Geometry: final body of the model. Coordinates: model frame, mm. Give positions to 0.01 mm unless a question says otherwise; leave off trailing zeros. Order: outer loops, then holes, each group sorted by start corner. A loop starts at its lowest first (then second) coordinate and runs counter-clockwise, first axis right, second up. Notation, with made-up numbers: (73, 77) - (131, 77) arc R34 ccw to (131, 109) - close; hole circle Ø3 at (1, -9). An arc over 180 degrees is marked (long way). Use one line per item in the form item = value.
Autodesk Inventor part; units mm, degrees
ref_plane "YZ Plane" through (0, 0, 0) normal (1, 0, 0) x (0, 1, 0)
ref_plane "XZ Plane" through (0, 0, 0) normal (0, 1, 0) x (-1, 0, 0)
ref_plane "XY Plane" through (0, 0, 0) normal (0, 0, 1) x (1, 0, 0)
ref_plane "Work Plane1" through (0, 0, 0) normal (0, 0, 1) x (1, 0, 0)
sketch "Sketch1" plane through (0, 0, 0) normal (0, 0, 1) x (1, 0, 0)
  line L0 (468.9048, -89.2586) -> (468.9048, 5.0009)
  arc A0 (468.9048, 5.0009) -> (465.7298, 8.1759) centre (465.7298, 5.0009) ccw
  line L1 (465.7298, 8.1759) -> (360.311, 8.1759)
  line L2 (458.2368, -92.4336) -> (458.2368, -2.4921)
  line L3 (458.2368, -2.4921) -> (357.136, -2.4921)
  arc A1 (360.311, 8.1759) -> (357.136, 5.0009) centre (360.311, 5.0009) ccw
  line L4 (357.136, 5.0009) -> (357.136, -89.2586)
  arc A2 (357.136, -89.2586) -> (360.311, -92.4336) centre (360.311, -89.2586) ccw
  line L5 (360.311, -92.4336) -> (465.7298, -92.4336)
  arc A3 (465.7298, -92.4336) -> (468.9048, -89.2586) centre (465.7298, -89.2586) ccw
  line L6 (468.9048, -89.2586) -> (468.9048, 5.0009)
  arc A4 (468.9048, 5.0009) -> (465.7298, 8.1759) centre (465.7298, 5.0009) ccw
  line L7 (465.7298, 8.1759) -> (360.311, 8.1759)
  circle A5 centre (437.65, 3.8619) radius 2.5844
  circle A6 centre (372.6092, -23.0789) radius 2.5844
  circle A7 centre (399.55, -88.1196) radius 2.5844
  circle A8 centre (464.5908, -61.1789) radius 2.5844
  circle A9 centre (372.6092, -88.1196) radius 2.413
  circle A10 centre (412.25, 3.8619) radius 2.413
  circle A11 centre (464.5908, -73.8789) radius 2.413
  circle A12 centre (464.5908, -48.4789) radius 2.413
  circle A13 centre (464.5908, -35.7789) radius 2.413
  circle A14 centre (374.15, 3.8619) radius 2.413
  circle A15 centre (386.85, 3.8619) radius 2.413
  arc A16 (365.5823, -19.7251) -> (365.5823, -17.8759) centre (362.2803, -18.8005) ccw
  line L8 (365.5823, -19.7251) -> (365.5823, -22.1025)
  line L9 (365.5823, -22.1025) -> (363.2049, -22.1025)
  arc A17 (361.3557, -22.1025) -> (363.2049, -22.1025) centre (362.2803, -18.8005) ccw
  line L10 (361.3557, -22.1025) -> (358.9783, -22.1025)
  line L11 (358.9783, -22.1025) -> (358.9783, -19.7251)
  arc A18 (358.9783, -17.8759) -> (358.9783, -19.7251) centre (362.2803, -18.8005) ccw
  line L12 (358.9783, -17.8759) -> (358.9783, -15.4985)
  line L13 (358.9783, -15.4985) -> (361.3557, -15.4985)
  arc A19 (363.2049, -15.4985) -> (361.3557, -15.4985) centre (362.2803, -18.8005) ccw
  line L14 (363.2049, -15.4985) -> (365.5823, -15.4985)
  line L15 (365.5823, -15.4985) -> (365.5823, -17.8759)
  circle A20 centre (424.95, 3.8619) radius 2.413
  arc A21 (358.9783, -64.5327) -> (358.9783, -66.3818) centre (362.2803, -65.4572) ccw
  line L16 (358.9783, -64.5327) -> (358.9783, -62.1552)
  line L17 (358.9783, -62.1552) -> (361.3557, -62.1552)
  arc A22 (363.2049, -62.1552) -> (361.3557, -62.1552) centre (362.2803, -65.4572) ccw
  line L18 (363.2049, -62.1552) -> (365.5823, -62.1552)
  line L19 (365.5823, -62.1552) -> (365.5823, -64.5327)
  arc A23 (365.5823, -66.3818) -> (365.5823, -64.5327) centre (362.2803, -65.4572) ccw
  line L20 (365.5823, -66.3818) -> (365.5823, -68.7592)
  line L21 (365.5823, -68.7592) -> (363.2049, -68.7592)
  arc A24 (361.3557, -68.7592) -> (363.2049, -68.7592) centre (362.2803, -65.4572) ccw
  line L22 (361.3557, -68.7592) -> (358.9783, -68.7592)
  line L23 (358.9783, -68.7592) -> (358.9783, -66.3818)
  circle A25 centre (464.5908, -86.5789) radius 2.413
  circle A26 centre (464.5908, -23.0789) radius 1.9844
  circle A27 centre (464.5908, 3.8619) radius 2.413
  circle A28 centre (361.45, 3.8619) radius 2.413
  circle A29 centre (418.6, -42.1289) radius 36.6
  circle A30 centre (437.65, -88.1196) radius 2.5844
  circle A31 centre (372.6092, -61.1789) radius 2.5844
  circle A32 centre (399.55, 3.8619) radius 2.5844
  circle A33 centre (418.6, -42.1289) radius 39.6368
  circle A34 centre (464.5908, 3.8619) radius 2.2479
  circle A35 centre (464.5908, -23.0789) radius 2.2479
  circle A36 centre (464.5908, -35.7789) radius 2.2479
  circle A37 centre (464.5908, -48.4789) radius 2.2479
  circle A38 centre (464.5908, -61.1789) radius 2.2479
  circle A39 centre (464.5908, -73.8789) radius 2.2479
  circle A40 centre (464.5908, -86.5789) radius 2.2479
  circle A41 centre (437.65, 3.8619) radius 2.2479
  circle A42 centre (424.95, 3.8619) radius 2.2479
  circle A43 centre (412.25, 3.8619) radius 2.2479
  circle A44 centre (399.55, 3.8619) radius 2.2479
  circle A45 centre (386.85, 3.8619) radius 2.2479
  circle A46 centre (374.15, 3.8619) radius 2.2479
  circle A47 centre (361.45, 3.8619) radius 2.2479
  point P0 (0, 0)
  point P1 (418.6, -2.4921)
  point P2 (458.2368, -42.1289)
  dimension "d0" = 10.668
  dimension "d2" = 4.4958
  dimension "d5" = 12.7
  dimension "d10" = 4.4958
  dimension "d13" = 12.7
extrude "Extrusion1" add sketch "Sketch1" along normal blind 1.5875 contours A3 L5 L2 L3 L4 A1 L1 A0 L0 | A33 L3 L2
fillet "Fillet1" radius 3.175 2 edges at (458.2368, -92.4336, 0.7938) (357.136, -2.4921, 0.7938)
properties part number "UnderGusset" material "Aluminum 6061"
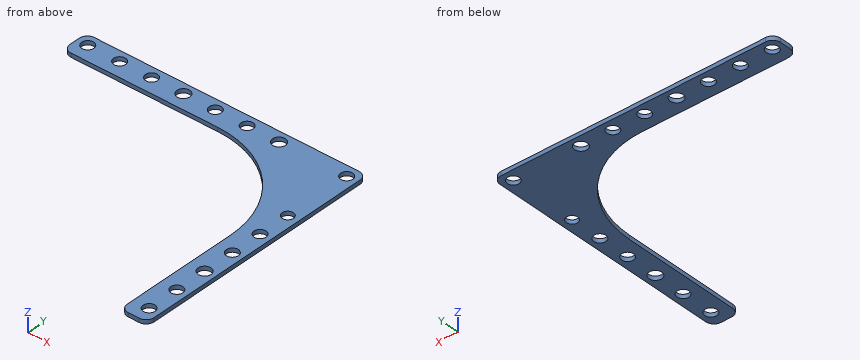
(1) Cut plane B-B on x = 399.55. Output: boundary loops of the cut face in (y, z), plus the area to 3 significant figures.
Computed values:
outline = (-2.49, 0) - (1.28, 0) - (1.28, 1.59) - (-2.49, 1.59) - close; (6.45, 0) - (8.18, 0) - (8.18, 1.59) - (6.45, 1.59) - close
area = 8.73 mm²
(2) Contact query for flat-ended pins moving along their axis: pin 1 Ø4.5 at (x, y) = (424.95, 3.86) entering from -Z; pin 2 Ø5 at (x, y) = (464.59, -23.08) entering from +Z; pin 3 Ø0.5 at (y, z) = (-66, 1) entering from -X; pin 4 Ø0.5 at (x, z) = (381, 1) entering from -Y. Output: stop coordinate, or through.
Computed values:
pin_1 = through
pin_2 = 1.59
pin_3 = 458.24
pin_4 = -2.49
(3) Ray query, line 1 along Y through (x, z) = (374.15, 0.7); line 2 along Y through (x, z) = (390, 0.85); line 3 along X through (y, z) = (-78, 0.65). Return the intervals inside material, ascending.
Computed values:
line_1 = -2.49 to 1.45, 6.27 to 8.18
line_2 = -2.49 to 8.18
line_3 = 458.24 to 468.9
(4) Cut plane D-D on y = -4. Output: boundary loops of the cut face in (x, z).
Computed values:
outline = (429.43, 0) - (468.9, 0) - (468.9, 1.59) - (429.43, 1.59) - close
(5) Cut plane C-C on y = -79.5. Output: boundary loops of the cut face in (x, z).
Computed values:
outline = (458.24, 0) - (468.9, 0) - (468.9, 1.59) - (458.24, 1.59) - close
(6) Cut plane A-A on x = 374.15. Output: boundary loops of the cut face in (y, z).
Computed values:
outline = (-2.49, 0) - (1.45, 0) - (1.45, 1.59) - (-2.49, 1.59) - close; (6.27, 0) - (8.18, 0) - (8.18, 1.59) - (6.27, 1.59) - close
